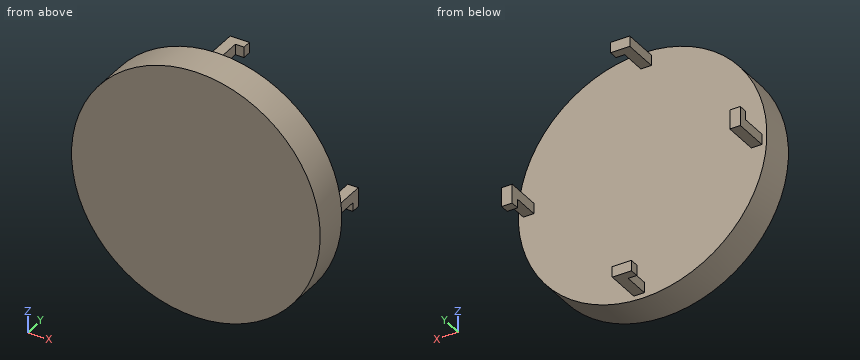
```python
from build123d import *

# Parameters (mm, degrees)
SKETCH1_R           = 45
BOSS_EXTRUDE1_DEPTH = 12.7
SKETCH2_W           = 3.81
SKETCH2_H           = 3.81
BOSS_EXTRUDE2_DEPTH = 12.7
SKETCH3_W           = 3.81
SKETCH3_H           = 3.175
BOSS_EXTRUDE3_DEPTH = 3.125
CIRPATTERN2_COUNT   = 4


with BuildPart() as part:
    # Sketch1 → Boss-Extrude1 (new body)
    with BuildSketch(Plane(origin=(0, 0, 0), x_dir=(1, 0, 0), z_dir=(0, 1, 0))):
        with Locations(Location((0, 0, 0), (0, 0, 270))):
            Circle(SKETCH1_R)
    extrude(amount=BOSS_EXTRUDE1_DEPTH)

    # Sketch2 → Boss-Extrude2 (add)
    with BuildSketch(Plane(origin=(0, 12.7, 0), x_dir=(1, 0, 0), z_dir=(0, 1, 0))):
        with Locations((-41.275, 1.27)):
            Rectangle(SKETCH2_W, SKETCH2_H)
    boss_extrude2 = extrude(amount=BOSS_EXTRUDE2_DEPTH)

    # Sketch3 → Boss-Extrude3 (add)
    with BuildSketch(Plane.XY.offset(0.635)):
        with Locations((-41.275, 23.8125)):
            Rectangle(SKETCH3_W, SKETCH3_H)
    boss_extrude3 = extrude(amount=BOSS_EXTRUDE3_DEPTH)

    # CirPattern2: Boss-Extrude2, Boss-Extrude3 ×4 about axis
    cirpattern2_axis = Axis((0, 0, 0), (0, 1, 0))
    add([boss_extrude2.rotate(cirpattern2_axis, i * 360 / CIRPATTERN2_COUNT) for i in range(1, CIRPATTERN2_COUNT)])
    add([boss_extrude3.rotate(cirpattern2_axis, i * 360 / CIRPATTERN2_COUNT) for i in range(1, CIRPATTERN2_COUNT)])


solid = part.part
```
Can you work these out from the model? Positions are in its coordinate system, mm. Round coordinates to 2 decimals unless told otherwise and drop trailing zeros. Order: outer loops, then holes, each group sorted by start corner. A loop starts at its lowest first (then second) coordinate and runs counter-clockwise, first axis right, second up. Notation, with made-up numbers: (8, -27.5) -> (44, -27.5) arc R23 cw to (44, 8.5) -> close; hole circle Ø10 at (-37, 27.5). An arc over 180 degrees is marked (long way). Return JSON: item names as keys, results as strings. Group by question number.
1. I need wall thicknesses on line 1 (X direction, y = 17, z = 0); line 2 (Y direction, x = 24.5, z = 21.5); line 3 (X direction, y = 10.75, z = 0). Which ranges of each line are inside material? Lowest first, please. Write a range as [from, to].
2. If we section it at A-A, the plane y = 23.75: Write out the boundary of the cut face in (x, z) (3 decimals), then the cut area to 3 significant figures.
3. If we section it at D-D, the plane x = -15.5: Write out the boundary of the cut face in (y, z), then the cut area to 3 significant figures.
4. If we section it at B-B, the plane y = 17.5: Write out the boundary of the cut face in (x, z) (3 decimals), then the cut area to 3 significant figures.
5. Will these pins go through, and if not, where does the flat tip stop? pin 1 (3.5 mm diameter, centred on y = 19.5, z = 0, fed in from -X); pin 2 (8 mm diameter, centred on x = -6.5, z = -14, fed in from +Y); pin 3 (2.5 mm diameter, centred on x = -41.5, y = 24, fed in from +Z).
6. If we section it at C-C, the plane z = 29: Write out the boundary of the cut face in (x, y).
Output values:
{
 "1": {"line 1": "[-43.18, -39.37], [39.37, 43.18]", "line 2": "[0, 12.7]", "line 3": "[-45, 45]"},
 "2": {"outline": "(-43.18, -3.175) -> (-39.37, -3.175) -> (-39.37, 3.76) -> (-43.18, 3.76) -> close; (-3.76, -43.18) -> (3.175, -43.18) -> (3.175, -39.37) -> (-3.76, -39.37) -> close; (-3.175, 39.37) -> (3.76, 39.37) -> (3.76, 43.18) -> (-3.175, 43.18) -> close; (39.37, -3.76) -> (43.18, -3.76) -> (43.18, 3.175) -> (39.37, 3.175) -> close", "area": "106 mm²"},
 "3": {"outline": "(0, -42.25) -> (12.7, -42.25) -> (12.7, 42.25) -> (0, 42.25) -> close", "area": "1,070 mm²"},
 "4": {"outline": "(-43.18, -3.175) -> (-39.37, -3.175) -> (-39.37, 0.635) -> (-43.18, 0.635) -> close; (-3.175, 39.37) -> (0.635, 39.37) -> (0.635, 43.18) -> (-3.175, 43.18) -> close; (-0.635, -43.18) -> (3.175, -43.18) -> (3.175, -39.37) -> (-0.635, -39.37) -> close; (39.37, -0.635) -> (43.18, -0.635) -> (43.18, 3.175) -> (39.37, 3.175) -> close", "area": "58.1 mm²"},
 "5": {"pin 1": "x = -43.18", "pin 2": "y = 12.7", "pin 3": "z = 3.76"},
 "6": {"outline": "(-34.41, 0) -> (34.41, 0) -> (34.41, 12.7) -> (-34.41, 12.7) -> close"}
}
